from build123d import *

# Parameters (mm, degrees)
F2_W     = 25.4
F2_H     = 4.7625
F3_DEPTH = 0.79375
F4_DEPTH = 0.79375
F5_R     = 0.635
F6_DEPTH = 25.4
F8_DEPTH = 2.54


with BuildPart() as f3:
    # F2 (on face) → F3 (new body, symmetric)
    with BuildSketch(Plane(origin=(0, 6.935504, -5.819579), x_dir=(-1, 0, 0), z_dir=(0, 0.766044, -0.642788))):
        with BuildLine():
            Line((-12.701223, 15.454063), (-12.701223, 2.754063))
            ThreePointArc((-12.701223, 2.754063), (-10.055389, -5.183437), (-3.176223, -9.945937))
            Line((-3.176223, -9.945937), (-0.001223, -9.945937))
            Line((-0.001223, -9.945937), (3.173777, -9.945937))
            ThreePointArc((3.173777, -9.945937), (10.052944, -5.183437), (12.698777, 2.754063))
            Line((12.698777, 2.754063), (12.698777, 15.454063))
            Line((12.698777, 15.454063), (-12.701223, 15.454063))
        make_face()
        with Locations((-0.001223, 17.835313)):
            Rectangle(F2_W, F2_H)
    extrude(amount=F3_DEPTH, both=True)

    # F0 (on Front) → F4 (join, symmetric)
    with BuildSketch(Plane.XZ):
        with BuildLine():
            Line((-12.7, 8.77501), (-12.7, -1.38499))
            ThreePointArc((-12.7, -1.38499), (-10.054167, -9.32249), (-3.175, -14.08499))
            Line((-3.175, -14.08499), (0, -14.08499))
            Line((0, -14.08499), (3.175, -14.08499))
            ThreePointArc((3.175, -14.08499), (10.054167, -9.32249), (12.7, -1.38499))
            Line((12.7, -1.38499), (12.7, 8.77501))
            Line((12.7, 8.77501), (-12.7, 8.77501))
        make_face()
    extrude(amount=F4_DEPTH, both=True)

    # F5 (on Right) → F6 (cut, symmetric)
    with BuildSketch(Plane.YZ):
        with Locations((0, -13.97)):
            Circle(F5_R)
    extrude(amount=F6_DEPTH, both=True, mode=Mode.SUBTRACT)

    # F7 (on face) → F8 (join)
    with BuildSketch(Plane.XZ.offset(0.79375)):
        with BuildLine():
            ThreePointArc((0, 4.8895), (1.032729, 5.317271), (1.4605, 6.35))
            ThreePointArc((1.4605, 6.35), (-1.032729, 7.382729), (0, 4.8895))
        make_face()
    extrude(amount=F8_DEPTH)


solid = f3.part
For this review, take the finished solid that the model builds, in its own axes (mm). A direction names the side the tool comes from. Round coordinates to 2 decimals unless told otherwise and drop trailing zeros. Loops run counter-clockwise (first coordinate to the right, second up) from the corner with the lowest first, then second, coordinate; pieces in that order, holes last. Notation, with made-up numbers: (73, 15) - (109, 15) arc R10 ccw to (109, 21) - close; hole circle Ø11 at (42.25, -37). An arc over 180 degrees is marked (long way). One line per item, written item: value. Start each with the question number.
Item 1: The part is to be moulded in two halves that separate along Y. For faces 1 (the flat face through (0.18, 19.94, 9.66)), 2 (the flat face through (0, -0.794, -2)), 3 (the cylindrical face through (10.126, 3.674, -9.724)), say which applies: +Y half, -Y half, draft (parallel to the pull), parting line (faces both ways), or undercut.
Item 2: Take a section at B-B (x = 8.75). Give the boundary of the cut face in (y, z) (3 decimals).
Item 3: For faces 4 (the cylindrical face through (-10.125, -0.011, -9.227)), 5 (the flat face through (0, 0, 8.775)), 6 (the flat face through (-12.699, 14, 3)), 7 (the cylindrical face through (9.98, -0.01, -9.42)), list the 3-axis set-ups (+Z, -Z, +X, -X, +Y, -Y) from which the entire face can be reached by the end or side of a thin tool; tool diameter is ignored.
Item 4: Take a section at D-D (x = 4.25). Give the boundary of the cut face in (y, z) (3 decimals), plus the area to 3 significant figures.
Item 5: For L1, parallel to Z at x = -2.5, y = 0 (3 decimals); L2, parallel to X at y = 9, z = -4.5; L3, parallel to Y at x = 2.75, z = -11.25 (3 decimals), list the stretches that pass through material, from the lowest coordinate up.
Item 6: Take a section at C-C (y = 0). Give the boundary of the cut face in (x, z) (3 decimals).
Item 7: Take a section at A-A (z = 5.5). Give the boundary of the cut face in (x, y).
Item 8: Clearance check with flat-ended pins moving along their axes: pin 1 Ø8 at (x, z) = (4.5, -7) entering from -Y; pin 2 Ø2 at (x, y) = (-7.5, 8) entering from -Z; pin 3 Ø1.7 at (x, y) = (-3.5, 0) entering from +Z (3 decimals). State where each tip first meets the part, or that it passes through.
Answer below:
1. face 1: +Y half
1. face 2: -Y half
1. face 3: undercut
2. outline: (-0.794, -10.814) - (0.794, -10.814) - (0.794, 8.775) - (-0.794, 8.775) - close; (2.036, -10.424) - (3.252, -11.444) - (20.539, 9.157) - (19.322, 10.177) - close
3. face 4: -Z, -X, -Y
3. face 5: +Z, +X, -X, -Y
3. face 6: +Z, -Z, -X, +Y, -Y
3. face 7: -Z, +X, -Y
4. outline: (-0.794, -13.721) - (-0.584, -13.721) arc R0.635 cw to (0.584, -13.721) - (0.794, -13.721) - (0.794, -13.175) - (1.384, -13.67) - (20.539, 9.157) - (19.322, 10.177) - (0.794, -11.904) - (0.794, 8.775) - (-0.794, 8.775) - close
4. area: 82.3 mm2
5. L1: z = -13.335 to 8.775
5. L2: x = -12.69 to 12.69
5. L3: y = -0.794 to 0.794, 1.343 to 3.415
6. outline: (-12.7, -1.385) arc R13.229 ccw to (-5.146, -13.335) - (5.146, -13.335) arc R13.229 ccw to (12.7, -1.385) - (12.7, 8.775) - (-12.7, 8.775) - close
7. outline: (-12.7, -0.79) - (-1.19, -0.79) - (-1.19, -3.33) - (1.19, -3.33) - (1.19, -0.79) - (12.7, -0.79) - (12.7, 0.79) - (-12.7, 0.79) - close; (-12.7, 15.4) - (12.7, 15.4) - (12.7, 17.47) - (-12.7, 17.47) - close
8. pin 1: stops at y = -0.79
8. pin 2: stops at z = -6.98
8. pin 3: stops at z = 8.775
